from build123d import *

# Parameters (mm, degrees)
SKETCH1_W           = 4
SKETCH1_H           = 5
BOSS_EXTRUDE1_DEPTH = 4
SKETCH2_W           = 20
SKETCH2_H           = 4
BOSS_EXTRUDE2_DEPTH = 4


with BuildPart() as part:
    # Sketch1 → Boss-Extrude1 (new body)
    with BuildSketch(Plane.XY):
        Polygon((-40, 30), (-50, 30), (-50, 25), (-50, 20), (-50, 15), (-50, 10), (-50, 5), (-50, -5), (-50, -10), (-50, -15), (-50, -20), (-50, -25), (-50, -30), (50, -30), (50, -25.221238938), (50, -25), (50, -20), (50, -15), (50, -10), (50, -5), (50, 0), (50, 5), (50, 6.10619469), (50, 10), (50, 15), (50, 20), (50, 25), (50, 30), (40, 30), (30, 30), (20, 30), (10, 30), (0, 30), (-10, 30), (-20, 30), (-30, 30), align=None)
        Polygon((-50, 10), (-50, 15), (-54, 15), (-54, 5), (-50, 5), align=None)
        with Locations((-52, 27.5)):
            Rectangle(SKETCH1_W, SKETCH1_H)
        Polygon((-50, -10), (-50, -5), (-54, -5), (-54, -15), (-50, -15), align=None)
        with Locations((-52, -27.5)):
            Rectangle(SKETCH1_W, SKETCH1_H)
        Polygon((54, 15), (50, 15), (50, 10), (50, 6.10619469), (50, 5), (54, 5), align=None)
        with Locations((52, 27.5)):
            Rectangle(SKETCH1_W, SKETCH1_H)
        Polygon((50, -10), (50, -15), (54, -15), (54, -5), (50, -5), align=None)
        Polygon((50, -25.221238938), (50, -30), (54, -30), (54, -25), (50, -25), align=None)
    extrude(amount=BOSS_EXTRUDE1_DEPTH)

    # Sketch2 → Boss-Extrude2 (add)
    with BuildSketch(Plane.XY.offset(4)):
        with Locations((0, 32)):
            Rectangle(SKETCH2_W, SKETCH2_H)
    extrude(amount=-BOSS_EXTRUDE2_DEPTH)


solid = part.part
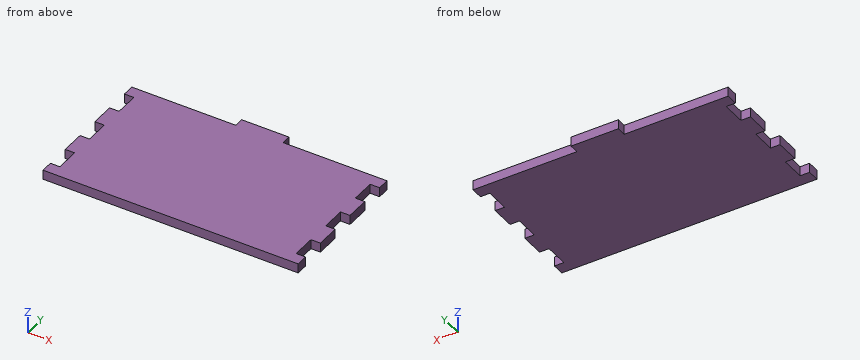
Model file for the job. Use its own axes, mm. Coordinates: 2 decimals unless noted, no trailing zeros. Write each loop counter-clockwise with the first axis right and the second up, starting at its lowest first coordinate (ties: lowest second). Pieces come first, ordered by that corner, then holes. Notation, with made-up numbers: (89, 41) - (98, 41) arc R13 ccw to (98, 59) - close; hole circle Ø7 at (77.5, 25.5). An arc over 180 degrees is marked (long way). Write each question's results on one line, items separated by ' | '. Start each with the question number.
1) Flat gauge pins, fed straight in: P1, Ø2, axis at y = 22, z = 2, coming from the +X side; P2, Ø2, axis at x = 51.5, z = 2.5, coming from the +Y side; P3, Ø1.2, axis at y = 32, z = 2, coming from the -X side. Where does each tip first touch, or does it go through?
2) Probe line 1 along Y through (x, z) = (-13, 1.1); line 2 along X through (y, z) = (-19.5, 2.5). List the from-to ranges inside material, lowest first. Write a range as from..to.
3) Cut at C-C (y = -20). Write the cut outline in (x, z).
4) Cut at B-B (x = -46). Write the cut outline in (y, z), then the cut area to 3 significant figures.
Returned:
1) P1: x = 50 | P2: y = 30 | P3: x = -10
2) line 1: -30..30 | line 2: -50..50
3) outline: (-50, 0) - (50, 0) - (50, 4) - (-50, 4) - close
4) outline: (-30, 0) - (30, 0) - (30, 4) - (-30, 4) - close | area: 240 mm^2
